Check sheet for the modelled part. Datum: model origin and axes. Units: mm. Round coordinates to 2 decimals unless told otherwise and drop trailing zeros. Order: outer loops, then holes, each group sorted by start corner. A loop starts at its lowest first (then second) coordinate and runs counter-clockwise, first axis right, second up. Notation, with made-up numbers: (-17, 4.25) -> (-2, 4.25) arc R16 cw to (-2, 24.25) -> close; hole circle Ø9 at (17.25, 64.5). An arc over 180 degrees is marked (long way). Answer as CSV lines item,"result". Start each with the question number.
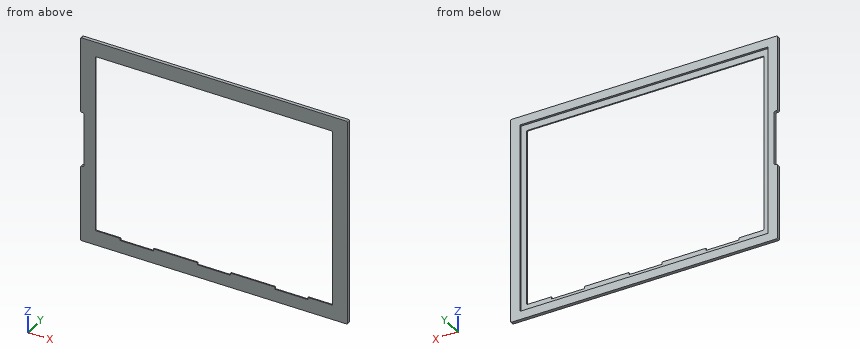
from build123d import *

# Parameters (mm, degrees)
SKETCH1_W           = 241.8
SKETCH1_H           = 188.8
SKETCH1_W_2         = 215
SKETCH1_H_2         = 162
BOSS_EXTRUDE1_DEPTH = 3
SKETCH2_W           = 225
SKETCH2_H           = 173.5
CUT_EXTRUDE1_DEPTH  = 2
SKETCH3_W           = 3
SKETCH3_H           = 50
CUT_EXTRUDE2_DEPTH  = 5
FILLET1_R           = 1
SKETCH4_W           = 30
SKETCH4_H           = 2
CUT_EXTRUDE3_DEPTH  = 4


with BuildPart() as part:
    # Sketch1 → Boss-Extrude1 (new body)
    with BuildSketch(Plane(origin=(0, 0, 0), x_dir=(1, 0, 0), z_dir=(0, 1, 0))):
        with Locations((120.9, 94.4)):
            Rectangle(SKETCH1_W, SKETCH1_H)
        with Locations((120.9, 94.4)):
            Rectangle(SKETCH1_W_2, SKETCH1_H_2, mode=Mode.SUBTRACT)
    extrude(amount=BOSS_EXTRUDE1_DEPTH)

    # Sketch2 → Cut-Extrude1 (cut)
    with BuildSketch(Plane(origin=(0, 3, 0), x_dir=(1, 0, 0), z_dir=(0, 1, 0))):
        with Locations((120.9, 94.4)):
            Rectangle(SKETCH2_W, SKETCH2_H)
    extrude(amount=-CUT_EXTRUDE1_DEPTH, mode=Mode.SUBTRACT)

    # Sketch3 → Cut-Extrude2 (cut)
    with BuildSketch(Plane(origin=(0, 3, 0), x_dir=(1, 0, 0), z_dir=(0, 1, 0))):
        with Locations((1.5, 94.4)):
            Rectangle(SKETCH3_W, SKETCH3_H)
    extrude(amount=-CUT_EXTRUDE2_DEPTH, mode=Mode.SUBTRACT)

    # Fillet1
    fillet1_edges = [part.edges().sort_by_distance(p)[0] for p in [
        (228.4, 0.5, -175.4),
        (13.4, 0.5, -175.4),
        (228.4, 0.5, -13.4),
        (13.4, 0.5, -13.4),
        (0, 1.5, -69.4),
        (0, 1.5, -119.4),
        (3, 1.5, -119.4),
        (3, 1.5, -69.4),
        (0, 1.5, -188.8),
        (241.8, 1.5, -188.8),
        (241.8, 1.5, 0),
        (0, 1.5, 0),
    ]]
    fillet(fillet1_edges, radius=FILLET1_R)

    # Sketch4 → Cut-Extrude3 (cut, through all)
    with BuildSketch(Plane.XZ):
        with Locations((50.9, -176.4)):
            Rectangle(SKETCH4_W, SKETCH4_H)
        with Locations((120.9, -176.4)):
            Rectangle(SKETCH4_W, SKETCH4_H)
        with Locations((190.9, -176.4)):
            Rectangle(SKETCH4_W, SKETCH4_H)
    extrude(amount=-CUT_EXTRUDE3_DEPTH, mode=Mode.SUBTRACT)


solid = part.part
1) Section check B-B on x = 122. Record the cut outline in (y, z), then the cut area to 3 significant figures.
2) Section check A-A on z = -143. Record the cut outline in (x, y).
3) Depth check by flat-ended pin: pin 1 Ø0.5 at (y, z) = (0.5, -113) entering from -X. Enter the tip coordinate at first touch or a pass-through.
4) Material ranges on line 1 along Z through (x, y) = (203, 0.5); line 2 along X through (y, z) = (1.3, -82); line 3 along Z through (x, y) = (60, 1.8), recorded low to high.
Solutions:
1,outline,"(0, -188.8) -> (3, -188.8) -> (3, -181.15) -> (1, -181.15) -> (1, -177.4) -> (0, -177.4) -> close; (0, -13.4) -> (1, -13.4) -> (1, -7.65) -> (3, -7.65) -> (3, 0) -> (0, 0) -> close"
1,area,"55.4 mm^2"
2,outline,"(0, 0) -> (13.4, 0) -> (13.4, 1) -> (8.4, 1) -> (8.4, 3) -> (0, 3) -> close; (228.4, 0) -> (241.8, 0) -> (241.8, 3) -> (233.4, 3) -> (233.4, 1) -> (228.4, 1) -> close"
3,pin 1,"stops at x = 3"
4,line 1,"z = -188.8 to -177.4, -13.4 to 0"
4,line 2,"x = 3 to 8.4, 233.4 to 241.8"
4,line 3,"z = -188.8 to -181.15, -7.65 to 0"
